```python
from build123d import *

# Parameters (mm, degrees)
F0_R        = 10
F1_DEPTH    = 10
F2_DEPTH    = 3
F2_FACE_R   = 17
F2_FACE_R_2 = 10
F4_DEPTH    = 10
F5_R        = 7.5
F6_DEPTH    = 10
F8_R        = 7.5
F9_DEPTH    = 10


with BuildPart() as f1:
    # F0 (on Top) → F1 (new body)
    with BuildSketch(Plane.XY):
        with BuildLine():
            Line((-36, -15), (-13.2287565553, -15))
            ThreePointArc((-13.2287565553, -15), (-20, 0), (-13.2287565553, 15))
            Line((-13.2287565553, 15), (-36, 15))
            Line((-36, 15), (-36, -15))
        make_face()
        with BuildLine():
            Line((-8, -15), (8, -15))
            ThreePointArc((8, -15), (14.5773797371, -8.7464278423), (17, 0))
            ThreePointArc((17, 0), (14.5773797371, 8.7464278423), (8, 15))
            Line((8, 15), (-8, 15))
            ThreePointArc((-8, 15), (-17, 0), (-8, -15))
        make_face()
        Circle(F0_R, mode=Mode.SUBTRACT)
        with BuildLine():
            Line((13.2287565553, -15), (36, -15))
            Line((36, -15), (36, 15))
            Line((36, 15), (13.2287565553, 15))
            ThreePointArc((13.2287565553, 15), (18.2287565553, 8.2287565553), (20, 0))
            ThreePointArc((20, 0), (18.2287565553, -8.2287565553), (13.2287565553, -15))
        make_face()
        with BuildLine():
            ThreePointArc((-13.2287565553, 15), (-20, 0), (-13.2287565553, -15))
            Line((-13.2287565553, -15), (-8, -15))
            ThreePointArc((-8, -15), (-17, 0), (-8, 15))
            Line((-8, 15), (-13.2287565553, 15))
        make_face()
        with BuildLine():
            Line((8, -15), (13.2287565553, -15))
            ThreePointArc((13.2287565553, -15), (18.2287565553, -8.2287565553), (20, 0))
            ThreePointArc((20, 0), (18.2287565553, 8.2287565553), (13.2287565553, 15))
            Line((13.2287565553, 15), (8, 15))
            ThreePointArc((8, 15), (14.5773797371, 8.7464278423), (17, 0))
            ThreePointArc((17, 0), (14.5773797371, -8.7464278423), (8, -15))
        make_face()
    extrude(amount=F1_DEPTH)

    # F0 (on Top) → F2 (join)
    with BuildSketch(Plane.XY):
        with BuildLine():
            Line((-8, -15), (8, -15))
            ThreePointArc((8, -15), (14.5773797371, -8.7464278423), (17, 0))
            ThreePointArc((17, 0), (14.5773797371, 8.7464278423), (8, 15))
            Line((8, 15), (-8, 15))
            ThreePointArc((-8, 15), (-17, 0), (-8, -15))
        make_face()
        Circle(F0_R, mode=Mode.SUBTRACT)
        with BuildLine():
            ThreePointArc((-8, -15), (0, -17), (8, -15))
            Line((8, -15), (-8, -15))
        make_face()
        with BuildLine():
            Line((-8, 15), (8, 15))
            ThreePointArc((8, 15), (0, 17), (-8, 15))
        make_face()
    extrude(amount=-F2_DEPTH)

    # F0 (on Top) + F2_face (on face) → F4 (join)
    with BuildSketch(Plane.XY):
        with BuildLine():
            ThreePointArc((-13.2287565553, -15), (0, -20), (13.2287565553, -15))
            Line((13.2287565553, -15), (8, -15))
            ThreePointArc((8, -15), (0, -17), (-8, -15))
            Line((-8, -15), (-13.2287565553, -15))
        make_face()
        with BuildLine():
            Line((8, -15), (13.2287565553, -15))
            ThreePointArc((13.2287565553, -15), (18.2287565553, -8.2287565553), (20, 0))
            ThreePointArc((20, 0), (18.2287565553, 8.2287565553), (13.2287565553, 15))
            Line((13.2287565553, 15), (8, 15))
            ThreePointArc((8, 15), (14.5773797371, 8.7464278423), (17, 0))
            ThreePointArc((17, 0), (14.5773797371, -8.7464278423), (8, -15))
        make_face()
        with BuildLine():
            Line((8, 15), (13.2287565553, 15))
            ThreePointArc((13.2287565553, 15), (0, 20), (-13.2287565553, 15))
            Line((-13.2287565553, 15), (-8, 15))
            ThreePointArc((-8, 15), (0, 17), (8, 15))
        make_face()
        with BuildLine():
            ThreePointArc((-13.2287565553, 15), (-20, 0), (-13.2287565553, -15))
            Line((-13.2287565553, -15), (-8, -15))
            ThreePointArc((-8, -15), (-17, 0), (-8, 15))
            Line((-8, 15), (-13.2287565553, 15))
        make_face()
        with BuildLine():
            ThreePointArc((-8, -15), (0, -17), (8, -15))
            Line((8, -15), (-8, -15))
        make_face()
        with BuildLine():
            Line((-8, 15), (8, 15))
            ThreePointArc((8, 15), (0, 17), (-8, 15))
        make_face()
    with BuildSketch(Plane(origin=(0, 0, -3), x_dir=(1, 0, 0), z_dir=(0, 0, -1))):
        Circle(F2_FACE_R)
        Circle(F2_FACE_R_2, mode=Mode.SUBTRACT)
    extrude(amount=F4_DEPTH, dir=(0, 0, 1))

    # F5 (on offset) → F6 (join)
    with BuildSketch(Plane.YZ.offset(36)):
        with BuildLine():
            Line((-15, 35), (-15, 0))
            Line((-15, 0), (15, 0))
            Line((15, 0), (15, 35))
            ThreePointArc((15, 35), (0, 50), (-15, 35))
        make_face()
        with Locations((0, 35)):
            Circle(F5_R, mode=Mode.SUBTRACT)
    extrude(amount=-F6_DEPTH)

    # F8 (on offset) → F9 (join)
    with BuildSketch(Plane(origin=(-36, 0, 0), x_dir=(0, -1, 0), z_dir=(-1, 0, 0))):
        with BuildLine():
            Line((-15, 35), (-15, 0))
            Line((-15, 0), (15, 0))
            Line((15, 0), (15, 35))
            ThreePointArc((15, 35), (0, 50), (-15, 35))
        make_face()
        with Locations((0, 35)):
            Circle(F8_R, mode=Mode.SUBTRACT)
    extrude(amount=-F9_DEPTH)


solid = f1.part
```
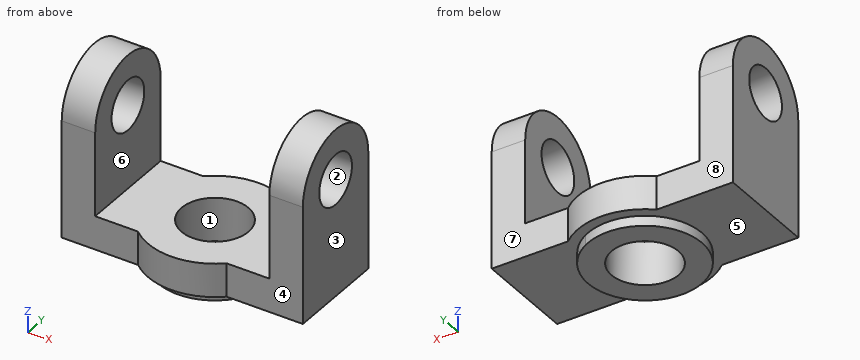
Design review of the part built by this model. Coordinates are the model's own, in mm. Face numbers are marked on the shaded views. A direction names the side the tool comes from. Coordinates: 2 decimals unless noted, no trailing zeros. Loops run counter-clockwise (first coordinate to the right, second up) from the corner with the lowest first, then second, coordinate; pieces in that order, holes last.
Q1. For pin 1 (11.5 mm diameter, centred on x = -23, z = 24.5, fed in from +Y); pin 2 (12 mm diameter, centred on x = 25.5, z = 25, fed in from -Y); pin 3 (1 mm diameter, centred on x = 27, y = 12.5, fed in from -Z), all flat-tipped, find the tip position at first contact; note any pin that passes through.
Reported:
pin 1: stops at y = 15
pin 2: stops at y = -15
pin 3: stops at z = 0
Q2. We need section D-D on x = -29. State the section outline as (y, z) points, and give its area (3 significant figures).
Reported:
outline: (-15, 0) - (15, 0) - (15, 35) arc R15 ccw to (-15, 35) - close; hole circle Ø15 at (0, 35)
area: 1,230 mm2
Q3. To check wall thickness, follow line 1 (Z direction, x = -29, y = 0); line 2 (X direction, y = 12, z = 29); line 3 (Z direction, x = -14, y = -9). State the ranges of each line that lie inside material, in increasing order.
Reported:
line 1: z = 0 to 27.5, 42.5 to 50
line 2: x = -36 to -26, 26 to 36
line 3: z = -3 to 10
Q4. We need section C-C on y = -1.5. State the section outline as (x, z) points, and give its area (3 significant figures).
Reported:
outline: (-36, 0) - (-16.93, 0) - (-16.93, -3) - (-9.89, -3) - (-9.89, 10) - (-26, 10) - (-26, 27.65) - (-36, 27.65) - close; (-36, 42.35) - (-26, 42.35) - (-26, 49.92) - (-36, 49.92) - close; (9.89, -3) - (16.93, -3) - (16.93, 0) - (36, 0) - (36, 27.65) - (26, 27.65) - (26, 10) - (9.89, 10) - close; (26, 42.35) - (36, 42.35) - (36, 49.92) - (26, 49.92) - close
area: 1,070 mm2
Q5. The part is to be moulded in two halves that separate along Y. For the marked faces 1, 2, 3 and 4, say which applies: +Y half, -Y half, draft (parallel to the pull), parting line (faces both ways), or undercut.
Reported:
face 1: undercut
face 2: undercut
face 3: draft
face 4: -Y half
Q6. We need section B-B on x = 0. State the section outline as (y, z) points, and give its area (3 significant figures).
Reported:
outline: (-20, 0) - (-17, 0) - (-17, -3) - (-10, -3) - (-10, 10) - (-20, 10) - close; (10, -3) - (17, -3) - (17, 0) - (20, 0) - (20, 10) - (10, 10) - close
area: 242 mm2
Q7. Tool access review of the marked faces 5, 6, 7 and 8: name each direction out of +Z, -Z, +X, -X, +Y, -Y from which nothing blocks a thin tool from reaching the whole face with its end or side.
Reported:
face 5: -Z
face 6: +Z, +Y, -Y
face 7: +Z, -Z, +X, +Y
face 8: +Z, -Z, -X, +Y
Q8. We need section A-A on z = 16. State the section outline as (x, y) points, and give its area (3 significant figures).
Reported:
outline: (-36, -15) - (-26, -15) - (-26, 15) - (-36, 15) - close; (26, -15) - (36, -15) - (36, 15) - (26, 15) - close
area: 600 mm2
